Build history of the part. All positions in model axes, mm. Give positions to 0.01 mm unless a question says otherwise; leave off trailing zeros. Order: outer loops, then holes, each group sorted by start corner. A loop starts at its lowest first (then second) coordinate and runs counter-clockwise, first axis right, second up. Notation, with made-up numbers: (45.25, 22) - (79.25, 22) arc R25 ccw to (79.25, 49) - close; hole circle Ø1 at (6, 43). An arc over 180 degrees is marked (long way). Write each question's results on one line, items separated by ' | '. Start each with the question number.
1) Drop a flat-ended pin along its axis: pin 1 Ø1.2 at (x, z) = (0, 22) entering from +Y. Give the stop position or say it passes through.
2) Cut at A-A on z = 76.6. List the corners of the cut face in (x, y).
3) Drill centre lines: line 1 along Z through (x, y) = (0, 0.25); line 2 along X through (y, z) = (0.5, 22); line 3 along X through (y, z) = (-0.15, 76.6). Where is each one in solid material? Low to high. Write a range as from..to.
4) Two-plate mould, pull along Z, no slides. Class faces 1 (the face through (0, 0.974, 45)), 2 (the face through (0, 0, 0)), 3 (the face through (-0.133, 0.014, 83.086)): +Z half, -Z half, draft (parallel to the pull), parting line (faces both ways), or undercut.
5) Cut at C-C on z = 22. List the corners of the cut face in (x, y), plus the area to 3 significant figures.
6) Cut at B-B on y = -0.2. List the corners of the cut face in (x, z), plus the area to 3 significant figures.
from build123d import *

# Parameters (mm, degrees)
SKETCH1_R               = 2.5
BOSS_EXTRUDE1_DEPTH     = 56
SKETCH2_W               = 4.604836256
SKETCH2_H               = 1.948199954
BOSS_EXTRUDE2_DEPTH     = 33.1
SKETCH3_R               = 1.022717979
CUT_EXTRUDE1_DEPTH      = 4.474099977
SKETCH4_R               = 0.75
CUT_EXTRUDE2_DEPTH      = 3.5
CUT_EXTRUDE2_DEPTH_BACK = 3.5
SKETCH5_OUTSIDE_W       = 24.876
SKETCH5_OUTSIDE_H       = 24.876
SKETCH5_OUTSIDE_W_2     = 4.604836256
SKETCH5_OUTSIDE_H_2     = 1.948199954
CUT_EXTRUDE3_DEPTH      = 90.1000001


with BuildPart() as part:
    # Sketch1 → Boss-Extrude1 (new body)
    with BuildSketch(Plane.XY):
        Circle(SKETCH1_R)
    extrude(amount=BOSS_EXTRUDE1_DEPTH)

    # Sketch2 → Boss-Extrude2 (add)
    with BuildSketch(Plane.XY.offset(56)):
        Rectangle(SKETCH2_W, SKETCH2_H)
    extrude(amount=BOSS_EXTRUDE2_DEPTH)

    # Sketch3 → Cut-Extrude1 (cut, through all)
    with BuildSketch(Plane(origin=(0, 0.974099977, 0), x_dir=(1, 0, 0), z_dir=(0, 1, 0))):
        with Locations((0, -76.6)):
            Circle(SKETCH3_R)
        with Locations((0, -84.1)):
            Circle(SKETCH3_R)
    extrude(amount=-CUT_EXTRUDE1_DEPTH, mode=Mode.SUBTRACT)

    # Sketch4 → Cut-Extrude2 (cut, two sides)
    with BuildSketch(Plane(origin=(0, 0, 0), x_dir=(1, 0, 0), z_dir=(0, 1, 0))) as cut_extrude2_sk:
        with Locations((0, -5)):
            Circle(SKETCH4_R)
        with Locations((0, -22)):
            Circle(SKETCH4_R)
    extrude(amount=CUT_EXTRUDE2_DEPTH, mode=Mode.SUBTRACT)
    extrude(cut_extrude2_sk.sketch, amount=-CUT_EXTRUDE2_DEPTH_BACK, mode=Mode.SUBTRACT)

    # Sketch5 outside → Cut-Extrude3 (cut, through all)
    with BuildSketch(Plane.XY.offset(89.1)):
        Rectangle(SKETCH5_OUTSIDE_W, SKETCH5_OUTSIDE_H)
        Rectangle(SKETCH5_OUTSIDE_W_2, SKETCH5_OUTSIDE_H_2, mode=Mode.SUBTRACT)
    extrude(amount=-CUT_EXTRUDE3_DEPTH, mode=Mode.SUBTRACT)


solid = part.part
Results:
1) pin 1: through
2) outline: (-2.3, -0.97) - (-1.02, -0.97) - (-1.02, 0.97) - (-2.3, 0.97) - close; (1.02, -0.97) - (2.3, -0.97) - (2.3, 0.97) - (1.02, 0.97) - close
3) line 1: 0..4.25, 5.75..21.25, 22.75..75.58, 77.62..83.08, 85.12..89.1 | line 2: -2.3..-0.75, 0.75..2.3 | line 3: -2.3..-1.02, 1.02..2.3
4) face 1: draft | face 2: -Z half | face 3: undercut
5) outline: (-2.3, -0.97) - (-0.75, -0.97) - (-0.75, 0.97) - (-2.3, 0.97) - close; (0.75, -0.97) - (2.3, -0.97) - (2.3, 0.97) - (0.75, 0.97) - close | area: 6.05 mm^2
6) outline: (-2.3, 0) - (2.3, 0) - (2.3, 89.1) - (-2.3, 89.1) - close; hole circle Ø2.05 at (0, 76.6); hole circle Ø2.05 at (0, 84.1); hole circle Ø1.5 at (0, 5); hole circle Ø1.5 at (0, 22) | area: 400 mm^2
